```python
from build123d import *

# Parameters (mm, degrees)
SKETCH1_W                                      = 306.05
SKETCH1_H                                      = 197.425
SKETCH1_R                                      = 10.775
BOSS_EXTRUDE1_DEPTH                            = 2.38125
SKETCH9_W                                      = 306.05
SKETCH9_H                                      = 2.38125
BOSS_EXTRUDE2_DEPTH                            = 3.175
SKETCH10_R                                     = 3.5
CUT_EXTRUDE1_DEPTH                             = 184.856965146
CSK_FOR_M3_FLAT_HEAD_MACHINE_SCREW1_AT_2_COUNT = 2
CSK_FOR_M3_FLAT_HEAD_MACHINE_SCREW1_AT_2_PITCH = 28.69
CSK_FOR_M3_FLAT_HEAD_MACHINE_SCREW1_AT_3_COUNT = 2
CSK_FOR_M3_FLAT_HEAD_MACHINE_SCREW1_AT_3_PITCH = 178.948509983
CSK_FOR_M3_FLAT_HEAD_MACHINE_SCREW1_AT_4_COUNT = 2
CSK_FOR_M3_FLAT_HEAD_MACHINE_SCREW1_AT_4_PITCH = 208.645558843
CSK_FOR_M3_FLAT_HEAD_MACHINE_SCREW1_AT_5_COUNT = 2
CSK_FOR_M3_FLAT_HEAD_MACHINE_SCREW1_AT_5_PITCH = 260.467597265
CSK_FOR_M3_FLAT_HEAD_MACHINE_SCREW1_AT_6_COUNT = 2
CSK_FOR_M3_FLAT_HEAD_MACHINE_SCREW1_AT_6_PITCH = 224.342
CSK_FOR_M3_FLAT_HEAD_MACHINE_SCREW1_AT_7_COUNT = 2
CSK_FOR_M3_FLAT_HEAD_MACHINE_SCREW1_AT_7_PITCH = 195.652
SKETCH13_R                                     = 6
CUT_EXTRUDE2_DEPTH                             = 184.856965146
SKETCH15_R                                     = 0.875
CUT_EXTRUDE3_DEPTH                             = 184.856965146


with BuildPart() as part:
    # Sketch1 → Boss-Extrude1 (new body)
    # profile 1 of 5: a face of its own
    with BuildSketch(Plane.XY):
        Rectangle(SKETCH1_W, SKETCH1_H)
        with Locations((-142.25, -87.9375)):
            Circle(SKETCH1_R, mode=Mode.SUBTRACT)
        with Locations((-130.25, -64.9375)):
            Circle(SKETCH1_R, mode=Mode.SUBTRACT)
    # profile 2 of 5: a face of its own
    with BuildSketch(Plane.XY):
        with Locations((-130.25, -64.9375)):
            Circle(SKETCH1_R)
    # profile 3 of 5: a face of its own
    with BuildSketch(Plane.XY):
        with Locations((-142.25, -87.9375)):
            Circle(SKETCH1_R)
    # profile 4 of 5: a face of its own
    with BuildSketch(Plane.XY):
        with BuildLine():
            ThreePointArc((-142.25, -98.7125), (-149.869075567, -95.556575567), (-153.025, -87.9375))
            Line((-153.025, -87.9375), (-153.025, -98.7125))
            Line((-153.025, -98.7125), (-142.25, -98.7125))
        make_face()
    # profile 5 of 5: a face of its own
    with BuildSketch(Plane.XY):
        Rectangle(SKETCH1_W, SKETCH1_H)
    extrude(amount=BOSS_EXTRUDE1_DEPTH)

    # Sketch9 → Boss-Extrude2 (add)
    with BuildSketch(Plane(origin=(0, 98.7125, 0), x_dir=(1, 0, 0), z_dir=(0, 1, 0))):
        with Locations((0, -1.190625)):
            Rectangle(SKETCH9_W, SKETCH9_H)
    extrude(amount=BOSS_EXTRUDE2_DEPTH)

    # Sketch10 → Cut-Extrude1 (cut, through all)
    with BuildSketch(Plane(origin=(0, 0, 0), x_dir=(-1, 0, 0), z_dir=(0, 0, -1))):
        with Locations((-134.610000066, 92.3625)):
            Circle(SKETCH10_R)
        with Locations((-124.450000066, 92.3625)):
            Circle(SKETCH10_R)
        with Locations((-143.817500066, -87.5375001)):
            Circle(SKETCH10_R)
        with Locations((-133.657500066, -87.5375001)):
            Circle(SKETCH10_R)
    cut_extrude1 = extrude(amount=-CUT_EXTRUDE1_DEPTH, mode=Mode.SUBTRACT)

    # Mirror1: Cut-Extrude1 across plane
    add(cut_extrude1.mirror(Plane(origin=(0, 0, 0), x_dir=(0, 0, 1), z_dir=(1, 0, 0))), mode=Mode.SUBTRACT)

    # Sketch12 → CSK for M3 Flat Head Machine Screw1 (revolve, cut)
    with BuildSketch(Plane(origin=(111.94, -83.7125, 0), x_dir=(0, 1, 0), z_dir=(1, 0, 0))):
        Polygon((0, 0), (0, 2.38125), (1.7, 2.38125), (1.7, 1.45), (3.15, 0), align=None)
    csk_for_m3_flat_head_machine_screw1 = revolve(axis=Axis((111.94, -83.7125, -6.35), (0, 0, 1)), mode=Mode.SUBTRACT)

    # CSK for M3 Flat Head Machine Screw1 at 2: CSK for M3 Flat Head Machine Screw1 ×2
    with Locations(*[(-i * CSK_FOR_M3_FLAT_HEAD_MACHINE_SCREW1_AT_2_PITCH, 0, 0) for i in range(1, CSK_FOR_M3_FLAT_HEAD_MACHINE_SCREW1_AT_2_COUNT)]):
        add(csk_for_m3_flat_head_machine_screw1, mode=Mode.SUBTRACT)

    # CSK for M3 Flat Head Machine Screw1 at 3: CSK for M3 Flat Head Machine Screw1 ×2
    with Locations(*[Vector(-0.17848709666869095, 0.9839422525345588, 0) * (i * CSK_FOR_M3_FLAT_HEAD_MACHINE_SCREW1_AT_3_PITCH) for i in range(1, CSK_FOR_M3_FLAT_HEAD_MACHINE_SCREW1_AT_3_COUNT)]):
        add(csk_for_m3_flat_head_machine_screw1, mode=Mode.SUBTRACT)

    # CSK for M3 Flat Head Machine Screw1 at 4: CSK for M3 Flat Head Machine Screw1 ×2
    with Locations(*[Vector(-0.5365079449598529, 0.8438952689729665, 0) * (i * CSK_FOR_M3_FLAT_HEAD_MACHINE_SCREW1_AT_4_PITCH) for i in range(1, CSK_FOR_M3_FLAT_HEAD_MACHINE_SCREW1_AT_4_COUNT)]):
        add(csk_for_m3_flat_head_machine_screw1, mode=Mode.SUBTRACT)

    # CSK for M3 Flat Head Machine Screw1 at 5: CSK for M3 Flat Head Machine Screw1 ×2
    with Locations(*[Vector(-0.7369054808176367, 0.6759957931384838, 0) * (i * CSK_FOR_M3_FLAT_HEAD_MACHINE_SCREW1_AT_5_PITCH) for i in range(1, CSK_FOR_M3_FLAT_HEAD_MACHINE_SCREW1_AT_5_COUNT)]):
        add(csk_for_m3_flat_head_machine_screw1, mode=Mode.SUBTRACT)

    # CSK for M3 Flat Head Machine Screw1 at 6: CSK for M3 Flat Head Machine Screw1 ×2
    with Locations(*[(-i * CSK_FOR_M3_FLAT_HEAD_MACHINE_SCREW1_AT_6_PITCH, 0, 0) for i in range(1, CSK_FOR_M3_FLAT_HEAD_MACHINE_SCREW1_AT_6_COUNT)]):
        add(csk_for_m3_flat_head_machine_screw1, mode=Mode.SUBTRACT)

    # CSK for M3 Flat Head Machine Screw1 at 7: CSK for M3 Flat Head Machine Screw1 ×2
    with Locations(*[(-i * CSK_FOR_M3_FLAT_HEAD_MACHINE_SCREW1_AT_7_PITCH, 0, 0) for i in range(1, CSK_FOR_M3_FLAT_HEAD_MACHINE_SCREW1_AT_7_COUNT)]):
        add(csk_for_m3_flat_head_machine_screw1, mode=Mode.SUBTRACT)

    # Sketch13 → Cut-Extrude2 (cut, through all)
    with BuildSketch(Plane(origin=(0, 0, 0), x_dir=(-1, 0, 0), z_dir=(0, 0, -1))):
        with Locations((-97.75, -79.7125001)):
            Circle(SKETCH13_R)
        with Locations((97.75, -79.7125001)):
            Circle(SKETCH13_R)
    extrude(amount=-CUT_EXTRUDE2_DEPTH, mode=Mode.SUBTRACT)

    # Sketch15 → Cut-Extrude3 (cut, through all)
    with BuildSketch(Plane(origin=(0, 0, 0), x_dir=(-1, 0, 0), z_dir=(0, 0, -1))):
        with Locations((86.25, 9.595433878)):
            Circle(SKETCH15_R)
        with Locations((-51.926, 57.596353878)):
            Circle(SKETCH15_R)
        with Locations((-17.426, 52.781407709)):
            Circle(SKETCH15_R)
        with Locations((-86.514, -43.220432291)):
            Circle(SKETCH15_R)
        with Locations((-121.014, -38.405486122)):
            Circle(SKETCH15_R)
        with Locations((-121.014, -19.469513878)):
            Circle(SKETCH15_R)
        with Locations((-86.514, -14.65456771)):
            Circle(SKETCH15_R)
        with Locations((-86.514, 4.780487709)):
            Circle(SKETCH15_R)
        with Locations((-121.014, 9.595433878)):
            Circle(SKETCH15_R)
        with Locations((-121.014, 28.536486122)):
            Circle(SKETCH15_R)
        with Locations((-86.514, 33.35143229)):
            Circle(SKETCH15_R)
        with Locations((-86.514, 52.781407709)):
            Circle(SKETCH15_R)
        with Locations((-121.014, 57.596353878)):
            Circle(SKETCH15_R)
        with Locations((-51.926, 28.536486122)):
            Circle(SKETCH15_R)
        with Locations((-17.426, 33.35143229)):
            Circle(SKETCH15_R)
        with Locations((-17.426, 4.780487709)):
            Circle(SKETCH15_R)
        with Locations((-51.926, 9.595433878)):
            Circle(SKETCH15_R)
        with Locations((-51.926, -19.469513878)):
            Circle(SKETCH15_R)
        with Locations((-17.426, -14.65456771)):
            Circle(SKETCH15_R)
        with Locations((-51.926, -38.405486122)):
            Circle(SKETCH15_R)
        with Locations((-17.426, -43.220432291)):
            Circle(SKETCH15_R)
        with Locations((17.162, -38.405486122)):
            Circle(SKETCH15_R)
        with Locations((17.162, -19.469513878)):
            Circle(SKETCH15_R)
        with Locations((51.662, -14.65456771)):
            Circle(SKETCH15_R)
        with Locations((17.162, 9.595433878)):
            Circle(SKETCH15_R)
        with Locations((51.662, 4.780487709)):
            Circle(SKETCH15_R)
        with Locations((51.662, 33.35143229)):
            Circle(SKETCH15_R)
        with Locations((17.162, 28.536486122)):
            Circle(SKETCH15_R)
        with Locations((17.162, 57.596353878)):
            Circle(SKETCH15_R)
        with Locations((51.662, 52.781407709)):
            Circle(SKETCH15_R)
        with Locations((86.25, 57.596353878)):
            Circle(SKETCH15_R)
        with Locations((120.75, 52.781407709)):
            Circle(SKETCH15_R)
        with Locations((86.25, 28.536486122)):
            Circle(SKETCH15_R)
        with Locations((120.75, 33.35143229)):
            Circle(SKETCH15_R)
        with Locations((51.662, -43.220432291)):
            Circle(SKETCH15_R)
        with Locations((86.25, -38.405486122)):
            Circle(SKETCH15_R)
        with Locations((86.25, -19.469513878)):
            Circle(SKETCH15_R)
        with Locations((120.75, 4.780487709)):
            Circle(SKETCH15_R)
        with Locations((120.75, -14.65456771)):
            Circle(SKETCH15_R)
        with Locations((120.75, -43.220432291)):
            Circle(SKETCH15_R)
    extrude(amount=-CUT_EXTRUDE3_DEPTH, mode=Mode.SUBTRACT)


solid = part.part
```
Here's how the part is built. I have some questions about the finished solid (model axes, mm). Coordinates: 2 decimals unless noted, no trailing zeros. Loops run counter-clockwise (first coordinate to the right, second up) from the corner with the lowest first, then second, coordinate; pieces in that order, holes last. Notation, with made-up numbers: (76.5, -39) - (101.5, -39) arc R24 cw to (101.5, -5) - close; hole circle Ø2 at (70, 76.25). An arc over 180 degrees is marked (long way). Return JSON: item names as keys, results as strings. Group by question number.
Item 1: We'd pull the mould along X, two halves only. Please class faces 1 (the face through (141.936, -84.586, 1.174)), 2 (the face through (-2, 0, 2.381)): +X half, -X half, draft (parallel to the pull), parting line (faces both ways), or undercut.
Item 2: If we section it at A-A on x = 97.75: Write out the boundary of the cut face in (y, z), and give its area (3 significant figures).
Item 3: I need wall thicknesses on line 1 (Y direction, x = -86.25, z = 1.45); line 2 (Y direction, x = -120.75, z = 1.3); line 3 (Y direction, x = 97.75, z = 0.6). Which ranges of each line are inside material? Lowest first, please. Write a range as from..to.
Item 4: Will this pin go through, and if not, where does the flat tip stop? P1, Ø1.4, axis at x = -51.66, y = 4.78, coming from the -Z side.
Calculated:
{
 "1": {"face 1": "undercut", "face 2": "draft"},
 "2": {"outline": "(-98.71, 0) - (-85.71, 0) - (-85.71, 2.38) - (-98.71, 2.38) - close; (-73.71, 0) - (101.89, 0) - (101.89, 2.38) - (-73.71, 2.38) - close", "area": "449 mm^2"},
 "3": {"line 1": "y = -98.71..-39.28, -37.53..-20.34, -18.59..8.72, 10.47..27.66, 29.41..56.72, 58.47..101.89", "line 2": "y = -98.71..-44.1, -42.35..-15.53, -13.78..3.91, 5.66..32.48, 34.23..51.91, 53.66..101.89", "line 3": "y = -98.71..-85.71, -73.71..101.89"},
 "4": {"P1": "passes through"}
}
